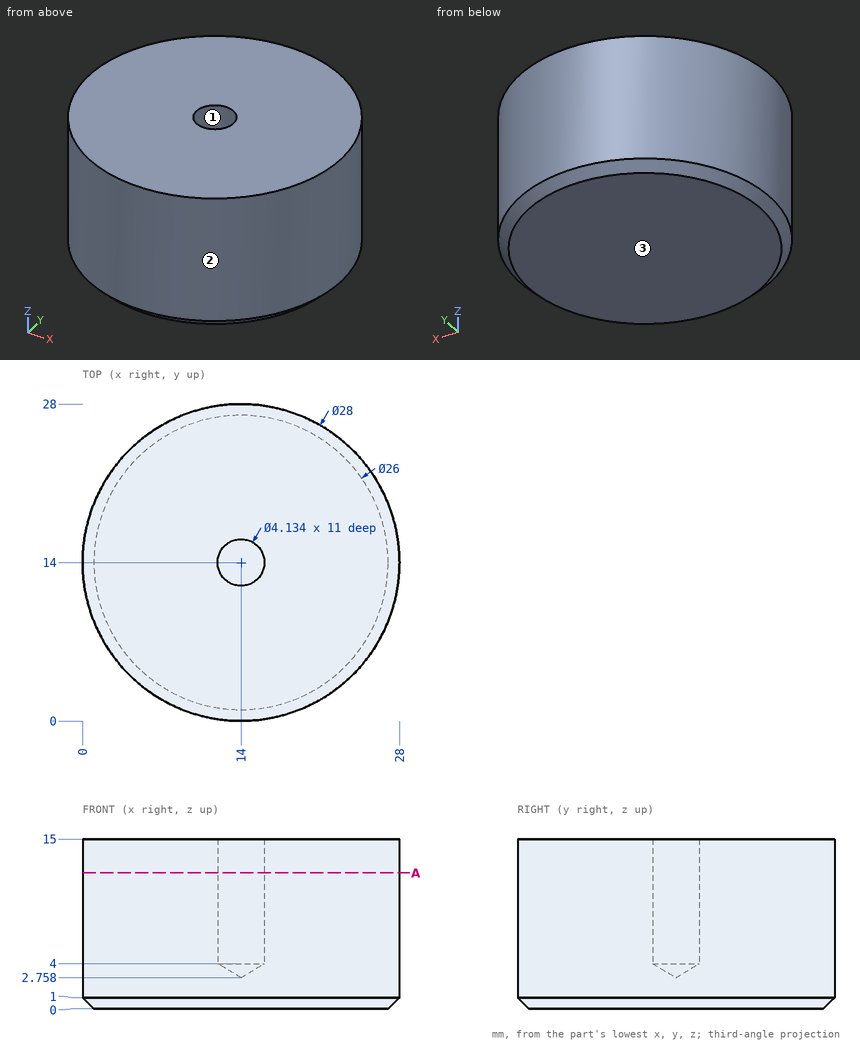
Drawing for the job (mm, zero at the part's lowest x, y, z). Give positions to 0.01 mm unless a question says otherwise; leave off trailing zeros. Write each loop counter-clockwise with the first axis right and the second up, starting at its lowest first coordinate (ties: lowest second). Pieces come first, ordered by that corner, then holes. Notation, with made-up numbers: (-16, -26) -> (10, -26) arc R14 cw to (10, -18) -> close; hole circle Ø9 at (-7.5, -33.5). An arc over 180 degrees is marked (long way). Put each result on its own line as item: value. Start each with the question number.
Item 1: Wall check: L1, parallel to X at y = 14, z = 11; L2, parallel to X at y = 12.25, z = 13.75. Give the ranges that are in metal, low to high. Write a range as [from, to].
Item 2: Cut at A-A (z = 12). List the corners of the cut face in (x, y).
Item 3: Pin check, flat tips, straight feed: pin 1 Ø1 at (x, z) = (19.5, 2) entering from -Y; pin 2 Ø1.5 at (y, z) = (5, 2) entering from -X; pin 3 Ø3 at (y, z) = (16, 11) entering from +X. Stop position of each tip, or through.
Item 4: Pull direction X, two halves, no side cores. Call the marked faces 1, 2 and 3: pulls with the +X half, pulls with the -X half, needs draft (parallel to the pull), parting line crosses it, or undercut.
Answer list:
1. L1: x = [0, 11.93], [16.07, 28]
1. L2: x = [0.11, 12.9], [15.1, 27.89]
2. outline: circle Ø28 at (14, 14); hole circle Ø4.13 at (14, 14)
3. pin 1: stops at y = 0.92
3. pin 2: stops at x = 2.69
3. pin 3: stops at x = 27.99
4. face 1: undercut
4. face 2: parting line crosses it
4. face 3: needs draft
